Here's how the part is built. I have some questions about the finished solid (model axes, mm). A direction names the side the tool comes from. Coordinates: 2 decimals unless noted, no trailing zeros. Write each loop counter-clockwise with the first axis right and the second up, starting at its lowest first coordinate (ties: lowest second). Pieces come first, ordered by that corner, then holes.
(1) Imagine slicing it at B-B, the plane y = 0. List the corners of the cut face in (x, z) for me, plus the area to 3 significant figures.
(2) Please list where these lines run through material, in increasing order: probe 1 along Y at (x, z) = (0, 7); probe 2 along Y at (x, z) = (24.5, 14); probe 3 along Y at (x, z) = (5.5, 14).
(3) Thinking about a two-plate mould opening in Z: for faces 1 (the flat face through (0, 1, 11)), 2 (the cylindrical face through (24.528, -32.176, 13.465)), 3 (the flat face through (21.311, -19, 8)), which applies, released by +Z, released by -Z, zero draft, split by the parting line, or undercut?
(4) For pin 1 Ø0.5 at (x, y) = (-13, -51.5) entering from -Z; pin 2 Ø3 at (x, y) = (-15.5, 0) entering from +Z, each with a flat end and sliding along its axis, tell me the tip position at first contact or that it passes through.
(5) Which directions (+Z, -Z, +X, -X, +Y, -Y) give clear straight access to the entire face, cutting with the end or side of a thin tool? Please do faces 4 (the flat face through (25, -17.5, 5)), 5 (the flat face through (-13.64, -2.39, 10.42)), 6 (the flat face through (21.311, 17, 8)).
(6) Imagine slicing it at C-C, the plane z = 6. State how many separate pieces and enclosed holes the cut face has, plus the area to 3 significant figures.
(7) Imagine slicing it at A-A, the plane x = 0. List the corners of the cut face in (y, z) for me, plus the area to 3 significant figures.
```python
from build123d import *

# Parameters (mm, degrees)
SKETCH1_W               = 42.62295082
SKETCH1_H               = 50
SKETCH1_R               = 2.677018134
BOSS_EXTRUDE1_DEPTH     = 16
SKETCH2_R               = 11
CUT_EXTRUDE2_DEPTH      = 11
SKETCH3_R               = 1.75
CUT_EXTRUDE3_DEPTH      = 10
CUT_EXTRUDE6_START      = -5
CUT_EXTRUDE6_DEPTH      = 32.540101042
SKETCH10_W              = 42.62295082
SKETCH10_H              = 16
BOSS_EXTRUDE2_DEPTH     = 16
SKETCH14_W              = 6
SKETCH14_H              = 13
CUT_EXTRUDE7_DEPTH      = 62.267576552
BOSS_EXTRUDE3_DEPTH     = 8
CUT_EXTRUDE9_DEPTH      = 8
SKETCH18_W              = 0.9
SKETCH18_H              = 4
SKETCH18_W_2            = 1.8
CUT_EXTRUDE10_DEPTH     = 10.2
CUT_EXTRUDE8_DEPTH      = 53.87875368
CUT_EXTRUDE8_DEPTH_BACK = 53.87875368
SKETCH15_R              = 1
CUT_EXTRUDE5_DEPTH      = 61.126222156
CUT_EXTRUDE5_DEPTH_BACK = 20
SKETCH6_W               = 9.034037672
SKETCH6_H               = 2.387531408
SKETCH20_W              = 8
SKETCH20_H              = 16
BOSS_EXTRUDE5_DEPTH     = 13
SKETCH21_W              = 8
SKETCH21_H              = 6
CUT_EXTRUDE11_DEPTH     = 13
SKETCH22_R              = 1
CUT_EXTRUDE12_DEPTH     = 53.87875368
SKETCH24_W              = 50.62295082
SKETCH24_H              = 5
BOSS_EXTRUDE6_DEPTH     = 15
SKETCH25_W              = 50.62295082
SKETCH25_H              = 15
BOSS_EXTRUDE7_DEPTH     = 11
SKETCH26_R              = 1
CUT_EXTRUDE13_DEPTH     = 10
SKETCH27_W              = 4
SKETCH27_H              = 1.8
CUT_EXTRUDE14_DEPTH     = 10.2
SKETCH29_W              = 20
SKETCH29_H              = 3.2
CUT_EXTRUDE15_DEPTH     = 5


with BuildPart() as part:
    # Sketch1 → Boss-Extrude1 (new body)
    with BuildSketch(Plane.XY):
        Rectangle(SKETCH1_W, SKETCH1_H)
        with Locations((-13, -15.25)):
            Circle(SKETCH1_R, mode=Mode.SUBTRACT)
        with Locations(Location((13, -15.25, 0), (0, 0, 180))):
            Circle(SKETCH1_R, mode=Mode.SUBTRACT)
        with Locations((13, 15.25)):
            Circle(SKETCH1_R, mode=Mode.SUBTRACT)
        with Locations(Location((-13, 15.25, 0), (0, 0, 180))):
            Circle(SKETCH1_R, mode=Mode.SUBTRACT)
    extrude(amount=BOSS_EXTRUDE1_DEPTH)

    # Sketch2 → Cut-Extrude2 (cut)
    with BuildSketch(Plane.XY):
        Circle(SKETCH2_R)
    extrude(amount=CUT_EXTRUDE2_DEPTH, mode=Mode.SUBTRACT)

    # Sketch3 → Cut-Extrude3 (cut)
    with BuildSketch(Plane(origin=(0, 0, 0), x_dir=(-1, 0, 0), z_dir=(0, 0, -1))):
        with Locations((-15, 0)):
            Circle(SKETCH3_R)
        with Locations(Location((15, 0, 0), (0, 0, 180))):
            Circle(SKETCH3_R)
    extrude(amount=-CUT_EXTRUDE3_DEPTH, mode=Mode.SUBTRACT)

    # Sketch9 → Cut-Extrude6 (cut, through all)
    with BuildSketch(Plane(origin=(0, 0, 0), x_dir=(-1, 0, 0), z_dir=(0, 0, -1)).offset(CUT_EXTRUDE6_START)):
        Polygon((-15, 3.175426481), (-17.75, 1.58771324), (-17.75, -1.58771324), (-15, -3.175426481), (-12.25, -1.58771324), (-12.25, 1.58771324), align=None)
        Polygon((12.25, 1.58771324), (15, 3.175426481), (17.75, 1.58771324), (17.75, -1.58771324), (15, -3.175426481), (12.25, -1.58771324), align=None)
    extrude(amount=-CUT_EXTRUDE6_DEPTH, mode=Mode.SUBTRACT)

    # Sketch10 → Boss-Extrude2 (add)
    with BuildSketch(Plane.XY):
        with Locations((0, -33)):
            Rectangle(SKETCH10_W, SKETCH10_H)
    extrude(amount=BOSS_EXTRUDE2_DEPTH)

    # Sketch14 → Cut-Extrude7 (cut, through all)
    with BuildSketch(Plane.ZY.offset(21.31147541)):
        with Locations((8, -34.5)):
            Rectangle(SKETCH14_W, SKETCH14_H)
    extrude(amount=-CUT_EXTRUDE7_DEPTH, mode=Mode.SUBTRACT)

    # Sketch16 → Boss-Extrude3 (add)
    with BuildSketch(Plane(origin=(21.31147541, 0, 0), x_dir=(0, 0, -1), z_dir=(1, 0, 0))):
        Polygon((-11, -28), (-8, -28), (-8, 25), (-16, 25), (-16, -28), align=None)
        Polygon((-8, 25), (-8, -28), (-5, -28), (0, -28), (0, 25), align=None)
    extrude(amount=BOSS_EXTRUDE3_DEPTH)

    # Sketch17 → Cut-Extrude9 (cut)
    with BuildSketch(Plane(origin=(29.31147541, 0, 0), x_dir=(0, 0, -1), z_dir=(1, 0, 0))):
        with BuildLine():
            ThreePointArc((-8, 17.675), (-9.175, 16.5), (-8, 15.325))
            Line((-8, 15.325), (-8, 17.675))
        make_face()
        with BuildLine():
            Line((-8, 17.675), (-8, 15.325))
            ThreePointArc((-8, 15.325), (-7.169149532, 15.669149532), (-6.825, 16.5))
            ThreePointArc((-6.825, 16.5), (-7.169149532, 17.330850468), (-8, 17.675))
        make_face()
        with BuildLine():
            ThreePointArc((-8, -18.325), (-9.175, -19.5), (-8, -20.675))
            Line((-8, -20.675), (-8, -18.325))
        make_face()
        with BuildLine():
            Line((-8, -18.325), (-8, -20.675))
            ThreePointArc((-8, -20.675), (-7.169149532, -20.330850468), (-6.825, -19.5))
            ThreePointArc((-6.825, -19.5), (-7.169149532, -18.669149532), (-8, -18.325))
        make_face()
    extrude(amount=-CUT_EXTRUDE9_DEPTH, mode=Mode.SUBTRACT)

    # Sketch18 → Cut-Extrude10 (cut)
    with BuildSketch(Plane(origin=(0, 0, 0), x_dir=(-1, 0, 0), z_dir=(0, 0, -1))):
        with Locations((-24.86147541, 16.5)):
            Rectangle(SKETCH18_W, SKETCH18_H)
        with Locations((-25.76147541, 16.5)):
            Rectangle(SKETCH18_W, SKETCH18_H)
        with Locations((-25.31147541, -19.5)):
            Rectangle(SKETCH18_W_2, SKETCH18_H)
    extrude(amount=-CUT_EXTRUDE10_DEPTH, mode=Mode.SUBTRACT)

    # Sketch15 → Cut-Extrude8 (cut, two sides: drawn at the far end of the back side and taken through both)
    with BuildSketch(Plane(origin=(0, 0, 0), x_dir=(-1, 0, 0), z_dir=(0, 0, -1)).offset(-CUT_EXTRUDE8_DEPTH_BACK)):
        with Locations(Location((16.31147541, -37.8, 0), (0, 0, 270))):
            Circle(SKETCH15_R)
        with Locations((16.31147541, -31.2)):
            Circle(SKETCH15_R)
    extrude(amount=CUT_EXTRUDE8_DEPTH + CUT_EXTRUDE8_DEPTH_BACK, mode=Mode.SUBTRACT)

    # Sketch6 → Cut-Extrude5 (cut, two sides: drawn at the far end of the back side and taken through both)
    with BuildSketch(Plane.XZ.offset(25).offset(-CUT_EXTRUDE5_DEPTH_BACK)):
        with Locations((0, 12.193765704)):
            Rectangle(SKETCH6_W, SKETCH6_H)
    extrude(amount=CUT_EXTRUDE5_DEPTH + CUT_EXTRUDE5_DEPTH_BACK, mode=Mode.SUBTRACT)

    # Sketch20 → Boss-Extrude5 (add)
    with BuildSketch(Plane(origin=(0, -28, 0), x_dir=(-1, 0, 0), z_dir=(0, -1, 0))):
        with Locations((-25.31147541, -8)):
            Rectangle(SKETCH20_W, SKETCH20_H)
    extrude(amount=BOSS_EXTRUDE5_DEPTH)

    # Sketch21 → Cut-Extrude11 (cut)
    with BuildSketch(Plane(origin=(0, -41, 0), x_dir=(-1, 0, 0), z_dir=(0, -1, 0))):
        with Locations((-25.31147541, -8)):
            Rectangle(SKETCH21_W, SKETCH21_H)
    extrude(amount=-CUT_EXTRUDE11_DEPTH, mode=Mode.SUBTRACT)

    # Sketch22 → Cut-Extrude12 (cut, through all)
    with BuildSketch(Plane(origin=(0, 0, 0), x_dir=(-1, 0, 0), z_dir=(0, 0, -1))):
        with Locations((-24.31147541, -37.8)):
            Circle(SKETCH22_R)
        with Locations((-24.31147541, -31.2)):
            Circle(SKETCH22_R)
    extrude(amount=-CUT_EXTRUDE12_DEPTH, mode=Mode.SUBTRACT)

    # Sketch24 → Boss-Extrude6 (add)
    with BuildSketch(Plane.XZ.offset(41)):
        with Locations((4, 2.5)):
            Rectangle(SKETCH24_W, SKETCH24_H)
    extrude(amount=BOSS_EXTRUDE6_DEPTH)

    # Sketch25 → Boss-Extrude7 (add)
    with BuildSketch(Plane.XY.offset(5)):
        with Locations((4, -48.5)):
            Rectangle(SKETCH25_W, SKETCH25_H)
    extrude(amount=BOSS_EXTRUDE7_DEPTH)

    # Sketch26 → Cut-Extrude13 (cut)
    with BuildSketch(Plane.XZ.offset(56)):
        with BuildLine():
            ThreePointArc((-15, 8), (-14, 7), (-13, 8))
            Line((-13, 8), (-15, 8))
        make_face()
        with BuildLine():
            Line((-15, 8), (-13, 8))
            ThreePointArc((-13, 8), (-14, 9), (-15, 8))
        make_face()
        with Locations(Location((22, 8, 0), (0, 0, 270))):
            Circle(SKETCH26_R)
    extrude(amount=-CUT_EXTRUDE13_DEPTH, mode=Mode.SUBTRACT)

    # Sketch27 → Cut-Extrude14 (cut)
    with BuildSketch(Plane(origin=(0, 0, 0), x_dir=(-1, 0, 0), z_dir=(0, 0, -1))):
        with Locations((-22.00147541, -52)):
            Rectangle(SKETCH27_W, SKETCH27_H)
        with Locations((14.00147541, -52)):
            Rectangle(SKETCH27_W, SKETCH27_H)
    extrude(amount=-CUT_EXTRUDE14_DEPTH, mode=Mode.SUBTRACT)

    # Sketch29 → Cut-Extrude15 (cut)
    with BuildSketch(Plane.XY.offset(16)):
        with Locations((4, -29.6)):
            Rectangle(SKETCH29_W, SKETCH29_H)
        Polygon((-6, -31.2), (-6, -32.875302663), (4, -34.5), (14, -32.875302663), (14, -31.2), align=None)
        Polygon((4, -34.5), (-6, -32.875302663), (-6, -36.124697337), align=None)
        with Locations((4, -39.4)):
            Rectangle(SKETCH29_W, SKETCH29_H)
        Polygon((14, -36.124697337), (4, -34.5), (-6, -36.124697337), (-6, -37.8), (14, -37.8), align=None)
        Polygon((14, -32.875302663), (4, -34.5), (14, -36.124697337), align=None)
    extrude(amount=-CUT_EXTRUDE15_DEPTH, mode=Mode.SUBTRACT)


solid = part.part
```
Recorded:
1. outline: (-21.31, 0) - (-16.75, 0) - (-16.75, 5) - (-17.75, 5) - (-17.75, 16) - (-21.31, 16) - close; (-13.25, 0) - (-11, 0) - (-11, 11) - (11, 11) - (11, 0) - (13.25, 0) - (13.25, 5) - (12.25, 5) - (12.25, 16) - (-12.25, 16) - (-12.25, 5) - (-13.25, 5) - close; (16.75, 0) - (29.31, 0) - (29.31, 16) - (17.75, 16) - (17.75, 5) - (16.75, 5) - close
1. area: 412 mm2
2. probe 1: y = -56 to -41, -28 to -11, 11 to 25
2. probe 2: y = -56 to -38.78, -36.82 to -32.18, -30.22 to 25
2. probe 3: y = -56 to -41, -28 to 25
3. face 1: released by -Z
3. face 2: zero draft
3. face 3: undercut
4. pin 1: stops at z = 10.2
4. pin 2: stops at z = 5
5. face 4: -Z
5. face 5: +Z
5. face 6: +X
6. separate pieces: 2
6. enclosed holes: 11
6. area: 2,890 mm2
7. outline: (-56, 0) - (-11, 0) - (-11, 11) - (-28, 11) - (-28, 5) - (-41, 5) - (-41, 16) - (-56, 16) - close; (-28, 13.39) - (-5, 13.39) - (-5, 11) - (11, 11) - (11, 0) - (25, 0) - (25, 16) - (-28, 16) - close
7. area: 856 mm2
